from build123d import *

# Parameters (mm, degrees)
F1_DEPTH = 30
F2_T     = -2
F3_R     = 5
F4_SIZE  = 1
F6_DEPTH = 0.4


# Not quite as in the source:
# - ends of sketch curves that miss each other by under 0.0002 mm in the source are joined


with BuildPart() as f1:
    # F0 (on Top) → F1 (new body)
    with BuildSketch(Plane.XY):
        with BuildLine():
            Line((38.72, 30.375), (-39.28, 30.375))
            ThreePointArc((-39.28, 30.375), (-46.3510678119, 27.4460678119), (-49.28, 20.375))
            Line((-49.28, 20.375), (-49.28, -16.125))
            ThreePointArc((-49.28, -16.125), (-46.3510678119, -23.1960678119), (-39.28, -26.125))
            Line((-39.28, -26.125), (38.72, -26.125))
            ThreePointArc((38.72, -26.125), (45.7910678119, -23.1960678119), (48.72, -16.125))
            Line((48.72, -16.125), (48.72, 20.375))
            ThreePointArc((48.72, 20.375), (45.7910678119, 27.4460678119), (38.72, 30.375))
        make_face()
    extrude(amount=F1_DEPTH)

    # F2
    f2_openings = [f1.faces().sort_by_distance(p)[0] for p in [
        (-0.28, 2.125, 30),
    ]]
    offset(amount=F2_T, openings=f2_openings)

    # F3
    f3_edges = [f1.edges().sort_by_distance(p)[0] for p in [
        (-0.28, -26.125, 0),
    ]]
    fillet(f3_edges, radius=F3_R)

    # F4
    f4_edges = [f1.edges().sort_by_distance(p)[0] for p in [
        (-0.28, -26.125, 30),
        (-46.351068, -23.196068, 30),
        (-49.28, 2.125, 30),
        (-46.351068, 27.446068, 30),
        (-0.28, 30.375, 30),
        (45.791068, 27.446068, 30),
        (48.72, 2.125, 30),
        (45.791068, -23.196068, 30),
    ]]
    chamfer(f4_edges, length=F4_SIZE)

    # F5 (on face) → F6 (cut)
    with BuildSketch(Plane(origin=(0, 0, 0), x_dir=(1, 0, 0), z_dir=(0, 0, -1))):
        with BuildLine():
            add(Edge.make_bspline(
                [(-8.093493, 9.19317), (-4.0467455, 12.8119), (2e-06, 12.8119), (4.0467495, 12.8119), (8.093497, 9.19317)],
                knots=[0, 0, 0, 0, 0.5, 1, 1, 1, 1], degree=3))
            Line((-8.093493, 9.19317), (0, 1.099674))
            Line((0, 1.099674), (8.093497, 9.19317))
        make_face()
        Polygon((-1.313547, 1e-06), (-9.40704, 8.093494), (-17.499982, 1e-06), (-9.40704, -8.092941), align=None)
        Polygon((17.499982, 1e-06), (9.406489, 8.093494), (1.312996, 1e-06), (9.406489, -8.092941), align=None)
        with BuildLine():
            Line((8.093495, -9.193168), (0, -1.099672))
            Line((0, -1.099672), (-8.093493, -9.193168))
            add(Edge.make_bspline(
                [(-8.093493, -9.193168), (-4.0467455, -12.811898), (2e-06, -12.811898), (4.0467495, -12.811898), (8.093495, -9.193168)],
                knots=[0, 0, 0, 0, 0.5, 1, 1, 1, 1], degree=3))
        make_face()
    extrude(amount=-F6_DEPTH, mode=Mode.SUBTRACT)


solid = f1.part
Can you work these out from the model? Positions are in its coordinate system, mm. A direction names the side the tool comes from. Round coordinates to 2 decimals unless told otherwise and drop trailing zeros. Loops run counter-clockwise (first coordinate to the right, second up) from the corner with the lowest first, then second, coordinate; pieces in that order, holes last. Notation, with made-up numbers: (83, 75.5) - (129, 75.5) arc R27 ccw to (129, 94.5) - close; hole circle Ø8 at (23.5, 67). An arc over 180 degrees is marked (long way). Write item = value, one per line. Start each with the question number.
(1) For faces 5 (the face through (5.416, -4.103, 0.197)), 6 (the face through (-45.838, -22.54, 29.826)), 7 (the face through (-1, -24.125, 16)), which set-ups out of +Z, -Z, +X, -X, +Y, -Y let a thin tool reach every point of the face, with its end or its side?
(2) If I drill on probe 1 along Y at (x, z) = (38, 14.5) (3 decimals); probe 2 along X at (y, z) = (-11.5, 8); probe 3 along Z at (x, y) = (38.5, 19.5), over which ranges is the centre line in solid material (lowest first)? Write a range as [from, to].
(3) For P1, Ø5, axis at x = -7.5, y = -3.5, coming from the -Z side; P2, Ø3.5, axis at x = -0.5, y = 6, coming from the -Z side, each with a flat end and sliding along its axis, tell me the tip position at first contact or that it passes through.
(4) If we mould it in two halves opening along Y, with no side actions, what happens to faces 1 (the face through (-13.4, -4.1, 0.2)), 2 (the face through (45.135, -22.683, 29.826)), 3 (the face through (-47.28, 2, 16)), 4 (the face through (-45.695, 26.933, 29.826))? For each: released by +Y, released by -Y, zero draft, split by the parting line, or undercut.
(5) If we section it at C-C (y = 17): Please give me the cut outline in (x, z), and give its area (3 significant figures).
(6) If we section it at D-D (x = -14): Please give me the cut outline in (y, z) (3 decimals), and give its area (3 significant figures).
(7) If we section it at A-A (x = -35): Please give me the cut outline in (y, z) (3 decimals).
(8) If we section it at B-B (z = 27.5): Please give me the cut outline in (x, y) (3 decimals), and give its area (3 significant figures).
Ans:
q1.face_5 = -Z
q1.face_6 = +Z, -X, -Y
q1.face_7 = +Z
q2.probe_1 = [-26.125, -24.125], [28.375, 30.375]
q2.probe_2 = [-49.28, -47.28], [46.72, 48.72]
q2.probe_3 = [0, 2]
q3.P1 = 0
q3.P2 = 0.4
q4.face_1 = undercut
q4.face_2 = released by -Y
q4.face_3 = undercut
q4.face_4 = released by +Y
q5.outline = (-49.28, 5) arc R5 ccw to (-44.28, 0) - (43.72, 0) arc R5 ccw to (48.72, 5) - (48.72, 29) - (47.72, 30) - (46.72, 30) - (46.72, 2) - (-47.28, 2) - (-47.28, 30) - (-48.28, 30) - (-49.28, 29) - close
q5.area = 296 mm²
q6.outline = (-26.125, 5) arc R5 ccw to (-21.125, 0) - (-3.5, 0) - (-3.5, 0.4) - (3.5, 0.4) - (3.5, 0) - (25.375, 0) arc R5 ccw to (30.375, 5) - (30.375, 29) - (29.375, 30) - (28.375, 30) - (28.375, 2) - (-24.125, 2) - (-24.125, 30) - (-25.125, 30) - (-26.125, 29) - close
q6.area = 210 mm²
q7.outline = (-26.125, 5) arc R5 ccw to (-21.125, 0) - (25.375, 0) arc R5 ccw to (30.375, 5) - (30.375, 29) - (29.375, 30) - (28.375, 30) - (28.375, 2) - (-24.125, 2) - (-24.125, 30) - (-25.125, 30) - (-26.125, 29) - close
q8.outline = (-49.28, -16.125) arc R10 ccw to (-39.28, -26.125) - (38.72, -26.125) arc R10 ccw to (48.72, -16.125) - (48.72, 20.375) arc R10 ccw to (38.72, 30.375) - (-39.28, 30.375) arc R10 ccw to (-49.28, 20.375) - close; hole (-47.28, -16.125) arc R8 ccw to (-39.28, -24.125) - (38.72, -24.125) arc R8 ccw to (46.72, -16.125) - (46.72, 20.375) arc R8 ccw to (38.72, 28.375) - (-39.28, 28.375) arc R8 ccw to (-47.28, 20.375) - close
q8.area = 571 mm²
